Input: part model. Units: mm. Frame: model coordinates. A direction names the side the tool comes from. Give positions to 0.01 mm unless a question says otherwise; leave off trailing zeros. Loops run counter-clockwise (first coordinate to the right, second up) from the corner with the lowest first, then second, coordinate; pieces in that order, holes last.
from build123d import *

# Parameters (mm, degrees)
SKETCH1_W                    = 27.305
SKETCH1_H                    = 8.4074
SKETCH1_R                    = 1.6129
BASE_PCB_DEPTH               = 1.905
SKETCH2_R                    = 3.429
SCREW_HEAD_UNSCREWED_DEPTH   = 2.032
SKETCH3_R                    = 2.921
THREADED_HOLE_BOSS_DEPTH     = 0.762
SKETCH4_R                    = 1.397
SCREW_STICKOUT_SCREWED_DEPTH = 0.889
SKETCH5_W                    = 0.508
SKETCH5_H                    = 1.4605
SKETCH5_W_2                  = 1.4605
SKETCH5_H_2                  = 0.508
F_2S_LIPO_MOUNTING_DEPTH     = 0.508


with BuildPart() as part:
    # Sketch1 → Base PCB (new body)
    with BuildSketch(Plane(origin=(0, 0, 0), x_dir=(1, 0, 0), z_dir=(0, 1, 0))):
        with Locations((13.6525, 4.2037)):
            Rectangle(SKETCH1_W, SKETCH1_H)
        with Locations(Location((3.2639, 4.2037, 0), (0, 0, 90))):
            Circle(SKETCH1_R, mode=Mode.SUBTRACT)
        with Locations(Location((19.3548, 4.2037, 0), (0, 0, 90))):
            Circle(SKETCH1_R, mode=Mode.SUBTRACT)
    extrude(amount=BASE_PCB_DEPTH)

    # Sketch2 → Screw Head (Unscrewed) (add)
    with BuildSketch(Plane(origin=(0, 1.905, 0), x_dir=(1, 0, 0), z_dir=(0, 1, 0))):
        with Locations(Location((11.30935, 4.2037, 0), (0, 0, 90))):
            Circle(SKETCH2_R)
    extrude(amount=SCREW_HEAD_UNSCREWED_DEPTH)

    # Sketch3 → Threaded Hole Boss (add)
    with BuildSketch(Plane.XZ):
        with Locations(Location((11.30935, -4.2037, 0), (0, 0, 90))):
            Circle(SKETCH3_R)
    extrude(amount=THREADED_HOLE_BOSS_DEPTH)

    # Sketch4 → Screw Stickout (Screwed) (add)
    with BuildSketch(Plane.XZ.offset(0.762)):
        with Locations(Location((11.30935, -4.2037, 0), (0, 0, 270))):
            Circle(SKETCH4_R)
    extrude(amount=SCREW_STICKOUT_SCREWED_DEPTH)

    # Sketch5 → 2s LiPo Mounting (cut)
    with BuildSketch(Plane(origin=(0, 3.937, 0), x_dir=(1, 0, 0), z_dir=(0, 1, 0))):
        with Locations((11.30935, 5.18795)):
            Rectangle(SKETCH5_W, SKETCH5_H)
        with Locations((10.3251, 4.2037)):
            Rectangle(SKETCH5_W_2, SKETCH5_H_2)
        with Locations((11.30935, 4.2037)):
            Rectangle(SKETCH5_W, SKETCH5_H_2)
        with Locations((11.30935, 3.21945)):
            Rectangle(SKETCH5_W, SKETCH5_H)
        with Locations((12.2936, 4.2037)):
            Rectangle(SKETCH5_W_2, SKETCH5_H_2)
    extrude(amount=-F_2S_LIPO_MOUNTING_DEPTH, mode=Mode.SUBTRACT)


solid = part.part
(1) Reachability of faces 4 (the flat face through (11, -1.651, -4)), 5 (the flat face through (13, -0.762, -5)) from +Z, -Z, +X, -X, +Y, -Y: full face, straight path, thin tool, end or side. Return the list, or none.
Values follow:
face 4: +Z, -Z, +X, -X, -Y
face 5: -Y
(2) Mould query, pull axis X, two halves, no side actions, for faces 1 (the flat face through (13, 1, -8.407)), 2 (the cylindrical face through (13.396, 2.907, -1.483)), 3 (the cylindrical face through (17.756, 0.939, -3.994)). Classes: +X half, -X half, draft (parallel to the pull), parting line (faces both ways), or undercut.
Values follow:
face 1: draft
face 2: parting line
face 3: undercut
(3) Pin query (flat end, axial travel): pin 1 Ø4 at (x, z) = (3, -3.5) entering from -Y; pin 2 Ø0.6 at (y, z) = (3.5, -5.5) entering from -X; pin 3 Ø0.6 at (x, y) = (12, 3.5) entering from +Z. Return the tip coordinate at first contact, or that it passes through.
Values follow:
pin 1: stops at y = 0
pin 2: stops at x = 8.03
pin 3: stops at z = -0.8
(4) Cut plane A-A (x = 4). Return the cut outline in (y, z) (3 decimals).
Values follow:
outline: (0, -8.407) - (1.905, -8.407) - (1.905, -5.639) - (0, -5.639) - close; (0, -2.769) - (1.905, -2.769) - (1.905, 0) - (0, 0) - close
(5) Ray query, probe 1 along X at (y, z) = (1.5, -3.25) (3 decimals); probe 2 along Y at (x, z) = (25, -0.25) (3 decimals); probe 3 along Y at (x, z) = (12.25, -1). Return the intervals inside material, ascending.
Values follow:
probe 1: x = 0 to 1.963, 4.565 to 18.054, 20.656 to 27.305
probe 2: y = 0 to 1.905
probe 3: y = 0 to 3.94
(6) Cut plane B-B (z = -3.5). Return the cut outline in (x, y) (1 decimal).
Values follow:
outline: (0, 0) - (1.8, 0) - (1.8, 1.9) - (0, 1.9) - close; (4.7, 0) - (8.5, 0) - (8.5, -0.8) - (10.1, -0.8) - (10.1, -1.7) - (12.5, -1.7) - (12.5, -0.8) - (14.1, -0.8) - (14.1, 0) - (17.9, 0) - (17.9, 1.9) - (14.7, 1.9) - (14.7, 3.9) - (11.6, 3.9) - (11.6, 3.4) - (11.1, 3.4) - (11.1, 3.9) - (8, 3.9) - (8, 1.9) - (4.7, 1.9) - close; (20.8, 0) - (27.3, 0) - (27.3, 1.9) - (20.8, 1.9) - close
(7) Cut plane D-D (x = 21.5). Return the cut outline in (y, z) (3 decimals).
Values follow:
outline: (0, -8.407) - (1.905, -8.407) - (1.905, 0) - (0, 0) - close
(8) Cut plane C-C (y = 0.55). Return the cut outline in (x, z) (3 decimals), and give its area (3 significant figures).
Values follow:
outline: (0, -8.407) - (27.305, -8.407) - (27.305, 0) - (0, 0) - close; hole circle Ø3.226 at (3.264, -4.204); hole circle Ø3.226 at (19.355, -4.204)
area: 213 mm2
